Input: part model. Units: mm. Frame: model coordinates. A direction names the side the tool comes from. Round coordinates to 2 decimals unless told otherwise and drop trailing zeros. Loops run counter-clockwise (first coordinate to the right, second up) from the corner with the lowest first, then second, coordinate; pieces in that order, holes last. Notation, with made-up numbers: M 24.5,81.25 L 30.5,81.25 A29 cw 30.5,105.25 Z; hole C 86.5,20.5 d8. An arc over 180 degrees is marked long. Put each result on its own line as item: value. Start each with the question number.
1) Section D-D on x = -8. Output: boundary loops of the cut face in (y, z).
2) Reachability of faces 1 (the face through (-17.96, 0.74, -8.6)), 2 (the face through (-2, 1.5, 2)) from +Z, -Z, +X, -X, +Y, -Y: full face, straight path, thin tool, end or side. Return the list, or none.
3) Section C-C on y = 4. Output: boundary loops of the cut face in (x, z).
4) Section B-B on z = -13. Output: boundary loops of the cut face in (x, y), plus the area to 3 significant figures.
5) Section A-A on x = 16.5. Output: boundary loops of the cut face in (y, z).
6) Pin query (flat end, axial travel): pin 1 (12 mm diameter, centred on x = 6, z = -2.5, fed in from +Y); pin 2 (6 mm diameter, centred on x = 6.5, y = 32.5, fed in from -Z). Return the tip coordinate at first contact, or that it passes through.
7) Draft query along Z for faces 3 (the face through (-21.41, 1, 10)), 4 (the face through (-18.12, 0.74, 14.21)), 5 (the face through (-2, 1, -17.411)), 6 (the face through (12.92, 0.74, -7.795)). Return one class per face: +Z half, -Z half, draft (parallel to the pull), parting line (faces both ways), or undercut.
8) Line query: probe 1 along Y at (x, z) = (4.5, -12); probe 2 along Z at (x, y) = (-2, 22). Output: solid intervals per line, ascending.
from build123d import *

# Parameters (mm, degrees)
SKETCH_1_W      = 40
SKETCH_1_H      = 41
SKETCH_1_R      = 1.75
EXTRUDE_1_DEPTH = 1.5
EXTRUDE_2_DEPTH = 1.5
FILLET_1_R      = 1.5


with BuildPart() as part:
    # 草图1 → 凸台-拉伸1 (new body)
    with BuildSketch(Plane(origin=(0, 0, 0), x_dir=(1, 0, 0), z_dir=(0, 1, 0))):
        with Locations((-1.409556314, -3.088737201)):
            Rectangle(SKETCH_1_W, SKETCH_1_H)
        with Locations(Location((-16.409556314, 9.411262799, 0), (0, 0, 270))):
            Circle(SKETCH_1_R, mode=Mode.SUBTRACT)
        with Locations(Location((-16.409556314, -14.588737201, 0), (0, 0, 270))):
            Circle(SKETCH_1_R, mode=Mode.SUBTRACT)
        with Locations(Location((13.590443686, 9.411262799, 0), (0, 0, 270))):
            Circle(SKETCH_1_R, mode=Mode.SUBTRACT)
        with Locations(Location((13.590443686, -14.588737201, 0), (0, 0, 270))):
            Circle(SKETCH_1_R, mode=Mode.SUBTRACT)
    extrude(amount=EXTRUDE_1_DEPTH)

    # 草图2 → 凸台-拉伸2 (add)
    with BuildSketch(Plane.XY.offset(23.588737201)):
        with BuildLine():
            Line((-21.409556314, 1.5), (-21.409556314, 26.02333316))
            ThreePointArc((-21.409556314, 26.02333316), (-1.409556314, 45), (18.590443686, 26.02333316))
            Line((18.590443686, 26.02333316), (18.590443686, 1.5))
            Line((18.590443686, 1.5), (18.590443686, 0))
            Line((18.590443686, 0), (-21.409556314, 0))
            Line((-21.409556314, 0), (-21.409556314, 1.5))
        make_face()
    extrude(amount=EXTRUDE_2_DEPTH)

    # 圆角1
    fillet_1_edges = [part.edges().sort_by_distance(p)[0] for p in [
        (-1.409556314, 0, 25.088737201),
        (-1.409556314, 1.5, 23.588737201),
    ]]
    fillet(fillet_1_edges, radius=FILLET_1_R)


solid = part.part
Geometry results:
1. outline: M 0,-17.41 L 1.5,-17.41 L 1.5,22.09 A1.5 cw 3,23.59 L 43.88,23.59 L 43.88,25.09 L 1.5,25.09 A1.5 ccw 0,23.59 Z
2. face 1: +Y, -Y
2. face 2: -Z, +X, -X, +Y
3. outline: M -21.41,23.59 L 18.59,23.59 L 18.59,25.09 L -21.41,25.09 Z
4. outline: M -21.41,0 L 18.59,0 L 18.59,1.5 L -21.41,1.5 Z
4. area: 60.0 mm²
5. outline: M 0,-17.41 L 1.5,-17.41 L 1.5,22.09 A1.5 cw 3,23.59 L 33.94,23.59 L 33.94,25.09 L 1.5,25.09 A1.5 ccw 0,23.59 Z
6. pin 1: stops at y = 1.5
6. pin 2: stops at z = 23.59
7. face 3: draft
7. face 4: undercut
7. face 5: -Z half
7. face 6: undercut
8. probe 1: y = 0 to 1.5
8. probe 2: z = 23.59 to 25.09
